Here's how the part is built. I have some questions about the finished solid (model axes, mm). Round coordinates to 2 decimals unless told otherwise and drop trailing zeros. Write each loop counter-clockwise with the first axis right and the second up, starting at its lowest first coordinate (ties: lowest second). Pieces come first, ordered by that corner, then holes. Notation, with made-up numbers: M 30,-36 L 41,-36 A24 ccw 41,-14 Z; hole C 62.25,-3 d3. An arc over 180 degrees is marked long. Write item = value, one per line. Start each with the question number.
(1) I need wall thicknesses on line 1 along Z through (x, y) = (-20, 1.25); line 2 along Z through (x, y) = (1.5, 8); line 3 along Z through (x, y) = (-21, 2.75). Which ranges of each line are inside material? Lowest first, please.
(2) If we mould it in two halves opening along X, with no side actions, what happens to faces 1 (the cylindrical face through (13.68, 9.86, -24.037)), 2 (the flat face through (-29.457, 9.86, 17.136)), 3 (the flat face through (0, 20, 7)), 4 (the flat face through (29.457, 9.86, -17.136))? For each: released by +X, released by -X, zero draft, split by the parting line, or undercut.
(3) I want a section at A-A (y = 16.25). List the corners of the cut face in (x, z) for me, and give its area (4 significant figures).
(4) I want a section at C-C (x = 0). List the corners of the cut face in (y, z) for me, and give its area (3 significant figures).
(5) I want a section at B-B (z = 0). List the corners of the cut face in (x, y) for me.
(6) Will these pins go through, and if not, where does the flat tip stop? pin 1 Ø5 at (x, y) = (-13.5, 13.5) entering from -Z; pin 2 Ø2 at (y, z) = (12, 16.5) entering from +X; pin 3 Ø1.5 at (x, y) = (-22.5, 14) entering from +Z.
(7) I want a section at D-D (z = 17). List the corners of the cut face in (x, y) for me.
```python
from build123d import *

# Parameters (mm, degrees)
SKETCH1_R           = 5
BOSS_EXTRUDE1_DEPTH = 20


with BuildPart() as part:
    # Sketch1 → Boss-Extrude1 (new body)
    with BuildSketch(Plane(origin=(0, 0, 0), x_dir=(1, 0, 0), z_dir=(0, 1, 0))):
        with BuildLine():
            Line((-7.979897677, 34.078163581), (7.979897677, 34.078163581))
            ThreePointArc((7.979897677, 34.078163581), (13.827467297, 23.949875898), (25.522606537, 23.949875898))
            Line((25.522606537, 23.949875898), (33.502504214, 10.128287683))
            ThreePointArc((33.502504214, 10.128287683), (27.654934594, 0), (33.502504214, -10.128287683))
            Line((33.502504214, -10.128287683), (25.522606537, -23.949875898))
            ThreePointArc((25.522606537, -23.949875898), (13.827467297, -23.949875898), (7.979897677, -34.078163581))
            Line((7.979897677, -34.078163581), (-7.979897677, -34.078163581))
            ThreePointArc((-7.979897677, -34.078163581), (-13.827467297, -23.949875898), (-25.522606537, -23.949875898))
            Line((-25.522606537, -23.949875898), (-33.502504214, -10.128287683))
            ThreePointArc((-33.502504214, -10.128287683), (-27.654934594, 0), (-33.502504214, 10.128287683))
            Line((-33.502504214, 10.128287683), (-25.522606537, 23.949875898))
            ThreePointArc((-25.522606537, 23.949875898), (-13.827467297, 23.949875898), (-7.979897677, 34.078163581))
        make_face()
        with Locations(Location((0, 0, 0), (0, 0, 270))):
            Circle(SKETCH1_R, mode=Mode.SUBTRACT)
    extrude(amount=BOSS_EXTRUDE1_DEPTH)


solid = part.part
```
Returned:
q1.line_1 = -22.39 to 22.39
q1.line_2 = -34.08 to -4.77, 4.77 to 34.08
q1.line_3 = -22.46 to 22.46
q2.face_1 = undercut
q2.face_2 = released by -X
q2.face_3 = zero draft
q2.face_4 = released by +X
q3.outline = M -33.5,-10.13 L -25.52,-23.95 A11.7 cw -7.98,-34.08 L 7.98,-34.08 A11.7 cw 25.52,-23.95 L 33.5,-10.13 A11.7 cw 33.5,10.13 L 25.52,23.95 A11.7 cw 7.98,34.08 L -7.98,34.08 A11.7 cw -25.52,23.95 L -33.5,10.13 A11.7 cw Z; hole C 0,0 d10
q3.area = 3,085 mm²
q4.outline = M 0,-34.08 L 20,-34.08 L 20,-5 L 0,-5 Z; M 0,5 L 20,5 L 20,34.08 L 0,34.08 Z
q4.area = 1,160 mm²
q5.outline = M -27.65,0 L -5,0 L -5,20 L -27.65,20 Z; M 5,0 L 27.65,0 L 27.65,20 L 5,20 Z
q6.pin_1 = -26.23
q6.pin_2 = 30.4
q6.pin_3 = 22.94
q7.outline = M -29.54,0 L 29.54,0 L 29.54,20 L -29.54,20 Z
